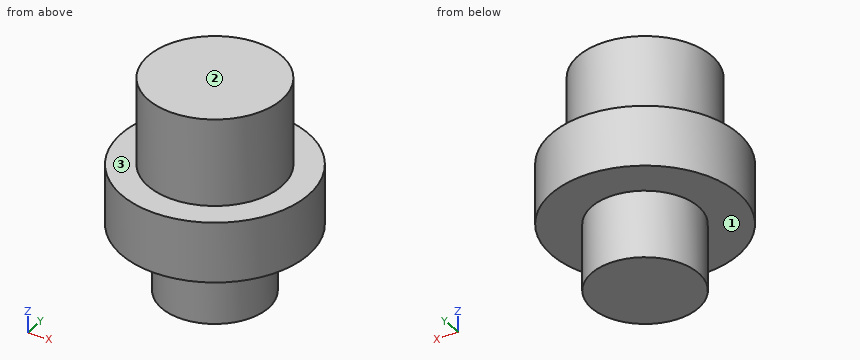
from build123d import *

# Parameters (mm, degrees)
CYLINDER001_R     = 7
CYLINDER001_DEPTH = 4.5
CYLINDER002_R     = 4
CYLINDER002_DEPTH = 5
CYLINDER_R        = 5
CYLINDER_DEPTH    = 6.5


with BuildPart() as cylinder:
    # Cylinder001 → Cylinder001 (new body)
    with BuildSketch(Plane.XY.offset(-4.5)):
        Circle(CYLINDER001_R)
    extrude(amount=CYLINDER001_DEPTH)


with BuildPart() as cylinder001:
    # Cylinder002 → Cylinder002 (new body)
    with BuildSketch(Plane.XY.offset(-9.5)):
        Circle(CYLINDER002_R)
    extrude(amount=CYLINDER002_DEPTH)


with BuildPart() as fusion:
    # Cylinder → Cylinder (new body)
    with BuildSketch(Plane.XY):
        Circle(CYLINDER_R)
    extrude(amount=CYLINDER_DEPTH)

    # Fusion: union Cylinder, Cylinder001
    add(cylinder.part)
    add(cylinder001.part)


solid = fusion.part
Design review of the part built by this model. Coordinates are the model's own, in mm. Face numbers are marked on the shaded views. A direction names the side the tool comes from. Coordinates: 2 decimals unless noted, no trailing zeros. Loops run counter-clockwise (first coordinate to the right, second up) from the corner with the lowest first, then second, coordinate; pieces in that order, holes last. Notation, with made-up numbers: (33.25, 53) -> (92.25, 53) arc R21 ccw to (92.25, 66) -> close; hole circle Ø5 at (68, 67.5). An arc over 180 degrees is marked (long way). Use a Markdown table: item, result. Add a question column.
Item 1: We need section A-A, the plane x = 0. Write out the cut boundary in (y, z), and give its area (3 significant figures).
Item 2: We need section D-D, the plane x = 4.75. Write out the cut boundary in (y, z).
Item 3: Machinability: for the marked faces 1, 2 and 3, which of the approach directions +Z, -Z, +X, -X, +Y, -Y give a long, thin tool a straight path to every point of the face, cutting with its end or side? Answer none if there is none.
Item 4: Clearance check with flat-ended pins moving along their axes: P1, Ø1.5, axis at x = 5, z = 4, coming from the +Y side; P2, Ø1.5, axis at x = -5.5, y = -1.5, coming from the -Z side; P3, Ø4, axis at x = 4.5, z = 3, coming from the -Y side; P4, Ø4, axis at y = 2, z = -5, coming from the -X side. State where each tip first meets the part, or that it passes through.
Item 5: We need section C-C, the plane z = -0.25. Write out the cut boundary in (x, y).
Item 6: Wall thickness on L1, parallel to Z at x = -3.5, y = 4; L2, parallel to X at y = 3, z = 5; L3, parallel to Y at x = -2.25, z = -5: over which ranges is each line inside the solid? List them lowest first. Write a range as from..to.
Numbers:
| question | item | result |
|---|---|---|
| 1 | outline | (-7, -4.5) -> (-4, -4.5) -> (-4, -9.5) -> (4, -9.5) -> (4, -4.5) -> (7, -4.5) -> (7, 0) -> (5, 0) -> (5, 6.5) -> (-5, 6.5) -> (-5, 0) -> (-7, 0) -> close |
| 1 | area | 168 mm^2 |
| 2 | outline | (-5.14, -4.5) -> (5.14, -4.5) -> (5.14, 0) -> (1.56, 0) -> (1.56, 6.5) -> (-1.56, 6.5) -> (-1.56, 0) -> (-5.14, 0) -> close |
| 3 | face 1 | -Z |
| 3 | face 2 | +Z, +X, -X, +Y, -Y |
| 3 | face 3 | +Z |
| 4 | P1 | stops at y = 2.63 |
| 4 | P2 | stops at z = -4.5 |
| 4 | P3 | stops at y = -4.33 |
| 4 | P4 | stops at x = -7 |
| 5 | outline | circle Ø14 at (0, 0) |
| 6 | L1 | z = -4.5..0 |
| 6 | L2 | x = -4..4 |
| 6 | L3 | y = -3.31..3.31 |
